The model under review builds one solid part; all positions refer to its coordinate system, in mm. Face numbers are marked on the shaded views. A direction names the side the tool comes from. Give positions to 0.01 mm unless a question says otherwise; leave off trailing zeros. Loops run counter-clockwise (first coordinate to the right, second up) from the corner with the lowest first, then second, coordinate; pieces in that order, holes last. Notation, with made-up numbers: (49.25, 18.25) - (60.25, 18.25) arc R16 ccw to (60.25, 26.25) - close; hole circle Ø5 at (59, 60.25). An arc over 180 degrees is marked (long way). Answer as a JSON object with one key per item and string values.
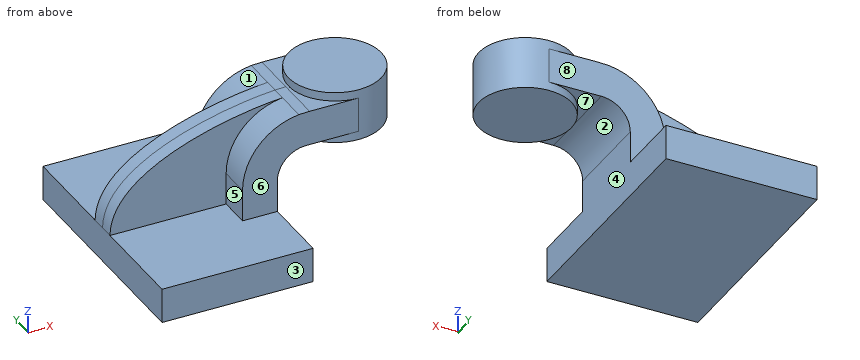
from build123d import *

# Parameters (mm, degrees)
F1_DEPTH = 63.5
F0_W     = 25.4
F0_H     = 19.05
F2_DEPTH = 25.4
F3_DEPTH = 7.9375


with BuildPart() as f1:
    # F0 (on Front) → F1 (new body, symmetric)
    with BuildSketch(Plane.XZ):
        Polygon((-41.275, 9.525), (-41.275, -9.525), (41.275, -9.525), (41.275, 9.525), (22.225, 9.525), align=None)
    extrude(amount=F1_DEPTH, both=True)

    # F0 (on Front) → F2 (join, symmetric)
    with BuildSketch(Plane.XZ):
        with BuildLine():
            Line((22.225, 9.525), (41.275, 9.525))
            Line((41.275, 9.525), (41.275, 27.0002))
            ThreePointArc((41.275, 27.0002), (45.92468, 38.22552), (57.15, 42.8752))
            Line((57.15, 42.8752), (60.325, 42.8752))
            Line((60.325, 42.8752), (60.325, 61.9252))
            Line((60.325, 61.9252), (58.905696, 61.9252))
            add(Edge.make_bspline(
                [(53.024491, 61.680682), (55.189714, 61.827395), (57.163409, 61.907619), (58.905696, 61.9252)],
                knots=[104.433612, 104.433612, 104.433612, 104.433612, 112.141058, 112.141058, 112.141058, 112.141058], degree=3))
            ThreePointArc((53.024491, 61.680682), (31.036411, 50.191494), (22.225, 27.0002))
            Line((22.225, 27.0002), (22.225, 9.525))
        make_face()
        with Locations((73.025, 52.4002)):
            Rectangle(F0_W, F0_H)
    extrude(amount=F2_DEPTH, both=True)

    # F0 (on Front) → F3 (join, symmetric)
    with BuildSketch(Plane.XZ):
        with BuildLine():
            add(Edge.make_bspline(
                [(-41.275, 9.525), (-40.815407, 45.497738), (23.686354, 59.692761), (53.024491, 61.680682)],
                knots=[0, 0, 0, 0, 104.433612, 104.433612, 104.433612, 104.433612], degree=3))
            Line((-41.275, 9.525), (22.225, 9.525))
            Line((22.225, 9.525), (22.225, 27.0002))
            ThreePointArc((22.225, 27.0002), (31.036411, 50.191494), (53.024491, 61.680682))
        make_face()
    extrude(amount=F3_DEPTH, both=True)

    # F0 (on Front) → F4 (revolve)
    with BuildSketch(Plane.XZ):
        Polygon((85.725, 66.675), (85.725, 61.9252), (85.725, 42.8752), (85.725, 38.1), (111.125, 38.1), (111.125, 66.675), align=None)
    revolve(axis=Axis((85.725, 0, 52.3875), (0, 0, 1)))


solid = f1.part
Q1. Clearance check with flat-ended pins moving along their axes: pin 1 Ø14 at (y, z) = (15.5, 17.5) entering from -X (3 decimals); pin 2 Ø14.5 at (x, y) = (75, 8) entering from -Z; pin 3 Ø18.5 at (y, z) = (9, 0.5) entering from +X (3 decimals). State where each tip first meets the part, or that it passes through.
Results:
{"pin 1": "stops at x = 22.225", "pin 2": "stops at z = 38.1", "pin 3": "stops at x = 41.275"}
Q2. To check wall thickness, follow probe 1 along Y at (x, z) = (74, 45.5); probe 2 along Z at (x, y) = (-14, 32.5) (3 decimals); probe 3 along X at (y, z) = (16.5, 4.5) (3 decimals). State the ranges of each line that lie inside material, in increasing order. Write a range as [from, to].
Results:
{"probe 1": "y = [-25.4, 25.4]", "probe 2": "z = [-9.525, 9.525]", "probe 3": "x = [-41.275, 41.275]"}
Q3. Consider section A-A, the plane y = -36. State the section outline as (x, z) points (3 decimals), plus the area to 3 significant figures.
Results:
{"outline": "(-41.275, -9.525) - (41.275, -9.525) - (41.275, 9.525) - (-41.275, 9.525) - close", "area": "1,570 mm^2"}
Q4. For the marked faces 4, 5, 6, 7 and 8, list the 3-axis set-ups (+Z, -Z, +X, -X, +Y, -Y) from which the entire face can be reached by the end or side of a thin tool; tool diameter is ignored.
Results:
{"face 4": "-Z, +X, +Y, -Y", "face 5": "+Z, -X, -Y", "face 6": "+Z, +X, -X, -Y", "face 7": "-Z", "face 8": "+Z, +X, -X, +Y"}
Q5. Consider section C-C, the plane z = 1. State the section outline as (x, y) points (3 decimals).
Results:
{"outline": "(-41.275, -63.5) - (41.275, -63.5) - (41.275, 63.5) - (-41.275, 63.5) - close"}
Q6. Consider section B-B, the plane x = 82.5. State the section outline as (y, z) points (3 decimals), plus the area to 3 significant figures.
Results:
{"outline": "(-25.4, 42.875) - (-25.194, 42.875) - (-25.194, 38.1) - (25.194, 38.1) - (25.194, 42.875) - (25.4, 42.875) - (25.4, 61.925) - (25.194, 61.925) - (25.194, 66.675) - (-25.194, 66.675) - (-25.194, 61.925) - (-25.4, 61.925) - close", "area": "1,450 mm^2"}
Q7. The part is to be moulded in two halves that separate along X. For the marked faces 1, 2 and 3, say which applies: +X half, -X half, draft (parallel to the pull), parting line (faces both ways), or undercut.
Results:
{"face 1": "-X half", "face 2": "undercut", "face 3": "draft"}
